Geometry check sheet. Reference: the model listing, model coordinates, mm. A direction names the side the tool comes from. Round coordinates to 2 decimals unless told otherwise and drop trailing zeros. Order: outer loops, then holes, each group sorted by start corner. A loop starts at its lowest first (then second) coordinate and runs counter-clockwise, first axis right, second up. Notation, with made-up numbers: (54, 54.25) -> (83, 54.25) arc R17 cw to (83, 84.25) -> close; hole circle Ø1 at (-10.75, -39.75). An arc over 180 degrees is marked (long way). Answer as a JSON object with one key per item and string values. Group by question number.
from build123d import *

# Parameters (mm, degrees)
SKETCH1_R           = 3.3734375
BOSS_EXTRUDE1_DEPTH = 3.175


with BuildPart() as part:
    # Sketch1 → Boss-Extrude1 (new body)
    with BuildSketch(Plane(origin=(0, 0, 0), x_dir=(0, 0, -1), z_dir=(1, 0, 0))):
        with BuildLine():
            Line((12.7, 0), (355.6, 0))
            ThreePointArc((355.6, 0), (364.580256121, 3.719743879), (368.3, 12.7))
            Line((368.3, 12.7), (368.3, 34.925))
            ThreePointArc((368.3, 34.925), (364.580256121, 43.905256121), (355.6, 47.625))
            Line((355.6, 47.625), (317.5, 47.625))
            ThreePointArc((317.5, 47.625), (308.519743879, 51.344743879), (304.8, 60.325))
            Line((304.8, 60.325), (304.8, 76.2))
            ThreePointArc((304.8, 76.2), (301.080256121, 85.180256121), (292.1, 88.9))
            Line((292.1, 88.9), (260.35, 88.9))
            ThreePointArc((260.35, 88.9), (251.369743879, 85.180256121), (247.65, 76.2))
            Line((247.65, 76.2), (247.65, 60.325))
            ThreePointArc((247.65, 60.325), (243.930256121, 51.344743879), (234.95, 47.625))
            Line((234.95, 47.625), (133.35, 47.625))
            ThreePointArc((133.35, 47.625), (124.369743879, 51.344743879), (120.65, 60.325))
            Line((120.65, 60.325), (120.65, 76.2))
            ThreePointArc((120.65, 76.2), (116.930256121, 85.180256121), (107.95, 88.9))
            Line((107.95, 88.9), (76.2, 88.9))
            ThreePointArc((76.2, 88.9), (67.219743879, 85.180256121), (63.5, 76.2))
            Line((63.5, 76.2), (63.5, 60.325))
            ThreePointArc((63.5, 60.325), (59.780256121, 51.344743879), (50.8, 47.625))
            Line((50.8, 47.625), (12.7, 47.625))
            ThreePointArc((12.7, 47.625), (3.719743879, 43.905256121), (0, 34.925))
            Line((0, 34.925), (0, 12.7))
            ThreePointArc((0, 12.7), (3.719743879, 3.719743879), (12.7, 0))
        make_face()
        with Locations((92.075, 76.2)):
            Circle(SKETCH1_R, mode=Mode.SUBTRACT)
        with Locations((276.225, 76.2)):
            Circle(SKETCH1_R, mode=Mode.SUBTRACT)
    extrude(amount=BOSS_EXTRUDE1_DEPTH)


solid = part.part
Item 1: Sectioned sample at B-B, the plane y = 63.5. Enter the section's corners in (x, z) (3 decimals).
Item 2: Sectioned sample at A-A, the plane x = 0.55. Enter the section's corners in (y, z) (3 decimals).
Item 3: Depth check by flat-ended pin: pin 1 Ø5.5 at (y, z) = (76.2, -276.225) entering from -X; pin 2 Ø1 at (x, z) = (1.5, -31) entering from +Y (3 decimals); pin 3 Ø1 at (x, y) = (1, 69.5) entering from +Z. Enter the tip coordinate at first touch or a pass-through.
Item 4: Sectioned sample at C-C, the plane z = -217.5. Enter the section's corners in (x, y) (3 decimals), then the cut area to 3 significant figures.
Item 5: Mould release check, pull along Y, two halves, no side actions. Record for faces 1 (the cylindrical face through (1.565, 51.444, -59.878)), 2 (the cylindrical face through (1.57, 78.48, -273.74)), 3 (the flat face through (0, 35, -182)), 4 (the cylindrical face through (1.57, 78.48, -89.59)): pulls with the +Y half, pulls with the -Y half, needs draft (parallel to the pull), parting line crosses it, or undercut.
Item 6: Thickness scan on L1, parallel to Y at x = 2.5, z = -215 (3 decimals); L2, parallel to Z at x = 1.7, y = 65; L3, parallel to Z at x = 0.45, y = 56. Record the ranges inside material, lowest first.
Item 7: Set-up check for faces 5 (the flat face through (3.175, 35, -182)), 6 (the cylindrical face through (1.565, 51.247, -124.469)): record each of +Z, -Z, +X, -X, +Y, -Y from which the full face is reachable in a straight line by a thin tool's end or side.
Result:
{
 "1": {"outline": "(0, -304.8) -> (3.175, -304.8) -> (3.175, -247.65) -> (0, -247.65) -> close; (0, -120.65) -> (3.175, -120.65) -> (3.175, -63.5) -> (0, -63.5) -> close"},
 "2": {"outline": "(0, -355.6) arc R12.7 ccw to (12.7, -368.3) -> (34.925, -368.3) arc R12.7 ccw to (47.625, -355.6) -> (47.625, -317.5) arc R12.7 cw to (60.325, -304.8) -> (76.2, -304.8) arc R12.7 ccw to (88.9, -292.1) -> (88.9, -260.35) arc R12.7 ccw to (76.2, -247.65) -> (60.325, -247.65) arc R12.7 cw to (47.625, -234.95) -> (47.625, -133.35) arc R12.7 cw to (60.325, -120.65) -> (76.2, -120.65) arc R12.7 ccw to (88.9, -107.95) -> (88.9, -76.2) arc R12.7 ccw to (76.2, -63.5) -> (60.325, -63.5) arc R12.7 cw to (47.625, -50.8) -> (47.625, -12.7) arc R12.7 ccw to (34.925, 0) -> (12.7, 0) arc R12.7 ccw to (0, -12.7) -> close; hole circle Ø6.747 at (76.2, -276.225); hole circle Ø6.747 at (76.2, -92.075)"},
 "3": {"pin 1": "passes through", "pin 2": "stops at y = 47.625", "pin 3": "stops at z = -63.5"},
 "4": {"outline": "(0, 0) -> (3.175, 0) -> (3.175, 47.625) -> (0, 47.625) -> close", "area": "151 mm2"},
 "5": {"face 1": "pulls with the +Y half", "face 2": "undercut", "face 3": "needs draft", "face 4": "undercut"},
 "6": {"L1": "y = 0 to 47.625", "L2": "z = -304.8 to -247.65, -120.65 to -63.5", "L3": "z = -305.56 to -246.89, -121.41 to -62.74"},
 "7": {"face 5": "+Z, -Z, +X, +Y, -Y", "face 6": "+X, -X, +Y"}
}
